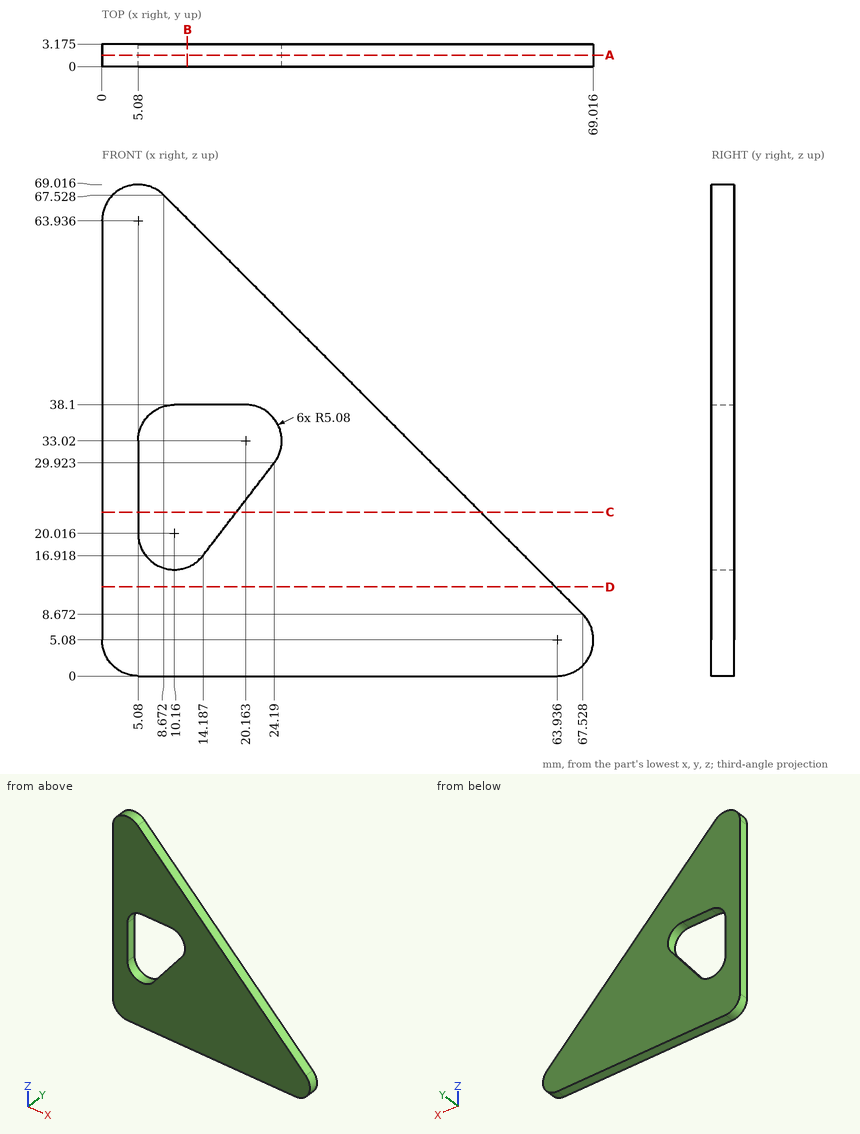
Job drawing, mm, ordinate dimensions from the low corner. One solid piece. Round coordinates to 2 decimals unless told otherwise and drop trailing zeros. Loops run counter-clockwise (first coordinate to the right, second up) from the corner with the lowest first, then second, coordinate; pieces in that order, holes last.
(1) Cut at B-B (x = 12). Give the cut face in (y, z) (1 decimal), plus the area to 3 significant figures.
(2) Cut at C-C (z = 23). Give the cut face in (x, y) (1 decimal).
(3) Drop a flat-ended pin along its axis: pin 1 (1.6 mm diameter, centred on y = 1.5, z = 29.5, fed in from +X). Give the stop position or say it passes through.
(4) Wall check: line 1 along X through (y, z) = (2.1, 24) (1 decimal); line 2 along Z through (x, y) = (17.5, 0.95) (1 decimal); line 3 along X through (y, z) = (2, 21) (1 decimal). Give the ranges that are in metal, low to high.
(5) Cut at A-A (y = 1.6). Give the cut face in (x, z) (1 decimal), plus the area to 3 significant figures.
(6) Cut at D-D (z = 12.5). Give the cut face in (x, y) (1 decimal).
Findings below:
1. outline: (0, 0) - (3.2, 0) - (3.2, 15.3) - (0, 15.3) - close; (0, 38.1) - (3.2, 38.1) - (3.2, 64.2) - (0, 64.2) - close
1. area: 131 mm2
2. outline: (0, 0) - (5.1, 0) - (5.1, 3.2) - (0, 3.2) - close; (18.9, 0) - (53.2, 0) - (53.2, 3.2) - (18.9, 3.2) - close
3. pin 1: stops at x = 47.5
4. line 1: x = 0 to 5.1, 19.6 to 52.2
4. line 2: z = 0 to 21.2, 38.1 to 58.7
4. line 3: x = 0 to 5.1, 17.3 to 55.2
5. outline: (0, 5.1) arc R5.1 ccw to (5.1, 0) - (63.9, 0) arc R5.1 ccw to (67.5, 8.7) - (8.7, 67.5) arc R5.1 ccw to (0, 63.9) - close; hole (5.1, 20) arc R5.1 ccw to (14.2, 16.9) - (24.2, 29.9) arc R5.1 ccw to (20.2, 38.1) - (10.2, 38.1) arc R5.1 ccw to (5.1, 33) - close
5. area: 2,490 mm2
6. outline: (0, 0) - (63.7, 0) - (63.7, 3.2) - (0, 3.2) - close
